Part model, mm, in its own coordinate system. A direction names the side the tool comes from. Give positions to 0.01 mm unless a question says otherwise; leave off trailing zeros. Order: outer loops, then holes, each group sorted by start corner. A loop starts at its lowest first (then second) coordinate and runs counter-clockwise, first axis right, second up. Notation, with made-up numbers: M 34.5,81 L 88.5,81 A32 cw 88.5,110 Z; hole C 33.25,19 d1. An arc over 180 degrees is marked long. Write each question's results on one line, items separated by ' | '. Start each with the question number.
from build123d import *

# Parameters (mm, degrees)
SKETCH1_R           = 5
BOSS_EXTRUDE1_DEPTH = 10
BOSS_EXTRUDE2_DEPTH = 10
SKETCH3_W           = 20
SKETCH3_H           = 20
SKETCH3_W_2         = 15
SKETCH3_H_2         = 15
BOSS_EXTRUDE3_DEPTH = 21
SKETCH4_W           = 50
SKETCH4_H           = 50
BOSS_EXTRUDE4_DEPTH = 3
SKETCH5_R           = 22.5
BOSS_EXTRUDE5_DEPTH = 75
SKETCH6_W           = 104.673759345
SKETCH6_H           = 11.076222709
BOSS_EXTRUDE6_DEPTH = 10


with BuildPart() as part:
    # Sketch1 → Boss-Extrude1 (new body)
    with BuildSketch(Plane(origin=(0, 0, 0), x_dir=(1, 0, 0), z_dir=(0, 1, 0))):
        with BuildLine():
            Line((0, 0), (30.876052193, 0))
            Line((30.876052193, 0), (30.876052193, -11.362717468))
            ThreePointArc((30.876052193, -11.362717468), (46.762190972, -21.786248919), (50, -3.063642105))
            Line((50, -3.063642105), (50, 0))
            Line((50, 0), (50, 50))
            Line((50, 50), (0, 50))
            Line((0, 50), (0, 0))
        make_face()
        with Locations(Location((42.238769661, -11.362717468, 0), (0, 0, 270))):
            Circle(SKETCH1_R, mode=Mode.SUBTRACT)
        with BuildLine():
            Line((9.874654059, 47.191553979), (24.296746366, 33.290272916))
            ThreePointArc((24.296746366, 33.290272916), (24.424993645, 26.799159409), (17.934255558, 26.653142217))
            Line((17.934255558, 26.653142217), (3.436266044, 40.475249935))
            ThreePointArc((3.436266044, 40.475249935), (3.288101967, 47.061421086), (9.874654059, 47.191553979))
        make_face(mode=Mode.SUBTRACT)
    extrude(amount=BOSS_EXTRUDE1_DEPTH)

    # Sketch2 → Boss-Extrude2 (add)
    with BuildSketch(Plane.XZ):
        Polygon((45, -5), (35, -5), (35, 0), (50, 0), (50, -15), (45, -15), align=None)
    extrude(amount=BOSS_EXTRUDE2_DEPTH)

    # Sketch3 → Boss-Extrude3 (add)
    with BuildSketch(Plane(origin=(0, 10, 0), x_dir=(1, 0, 0), z_dir=(0, 1, 0))):
        with Locations((10, 10)):
            Rectangle(SKETCH3_W, SKETCH3_H)
        with Locations((42.5, 42.5)):
            Rectangle(SKETCH3_W_2, SKETCH3_H_2)
    extrude(amount=BOSS_EXTRUDE3_DEPTH)

    # Sketch4 → Boss-Extrude4 (add)
    with BuildSketch(Plane(origin=(0, 31, 0), x_dir=(1, 0, 0), z_dir=(0, 1, 0))):
        with Locations((25, 25)):
            Rectangle(SKETCH4_W, SKETCH4_H)
    extrude(amount=BOSS_EXTRUDE4_DEPTH)

    # Sketch5 → Boss-Extrude5 (add)
    with BuildSketch(Plane(origin=(0, 34, 0), x_dir=(1, 0, 0), z_dir=(0, 1, 0))):
        with Locations(Location((25, 25, 0), (0, 0, 270))):
            Circle(SKETCH5_R)
    extrude(amount=BOSS_EXTRUDE5_DEPTH)

    # Sketch6 → Boss-Extrude6 (add)
    with BuildSketch(Plane(origin=(0, 109, 0), x_dir=(1, 0, 0), z_dir=(0, 1, 0))):
        with Locations((-23.301664344, 22.675113634)):
            Rectangle(SKETCH6_W, SKETCH6_H)
    extrude(amount=BOSS_EXTRUDE6_DEPTH)


solid = part.part
(1) Saw through at B-B on x = 13. Give the cut face in (y, z).
(2) Tool access for faces 4 (the flat face through (25, 31, -25)), 5 (the flat face through (16.985, 4.93, -40.338)), 6 (the flat face through (29.035, 114, -23)): list every direction of +Z, -Z, +X, -X, +Y, -Y with a clear straight run to the whole face (end or side of a thin tool).
(3) Saw through at C-C on x = -47. Give the cut face in (y, z), plus the area to 3 significant figures.
(4) Drop flat-ended pins along their axis: P1, Ø3, axis at x = 40, y = -4, coming from the -Z side; P2, Ø12, axis at y = 35.5, z = -38, coming from the -X side; P3, Ø11, axis at y = 112.5, z = -20.5, coming from the +X side; P4, Ø12, axis at x = -38.5, y = 99, coming from the -Z side. Give the stop position or say it passes through.
(5) Saw through at D-D on y = 62. Give the cut face in (x, z).
(6) Saw through at A-A on y = 28. Give the cut face in (x, z).
(7) Pull direction Z, two halves, no side cores. Call faces 1 (the flat face through (26, 0, -22)), 2 (the flat face through (40, -5, -5)), 3 (the cylindrical face through (24.49, 4.93, -26.87)): +Z half, -Z half, draft (parallel to the pull), parting line (faces both ways), or undercut.
(8) Probe L1, parallel to Y at x = 23, z = -2; L2, parallel to X at y = 8, z = -5.5; L3, parallel to Y at x = -46.5, z = -28. List the from-to ranges inside material, lowest first.
Taken from the geometry:
1) outline: M 0,-50 L 10,-50 L 10,-44.18 L 0,-44.18 Z; M 0,-31.36 L 10,-31.36 L 10,-20 L 31,-20 L 31,-50 L 34,-50 L 34,-44.03 L 109,-44.03 L 109,-28.21 L 119,-28.21 L 119,-17.14 L 109,-17.14 L 109,-5.97 L 34,-5.97 L 34,0 L 0,0 Z
2) face 4: none | face 5: -Y | face 6: +Z, -Z, +X, +Y
3) outline: M 109,-28.21 L 119,-28.21 L 119,-17.14 L 109,-17.14 Z | area: 111 mm²
4) P1: stops at z = -5 | P2: stops at x = 0 | P3: stops at x = 47.5 | P4: passes through
5) outline: C 25,-25 d45
6) outline: M 0,-20 L 20,-20 L 20,0 L 0,0 Z; M 35,-50 L 50,-50 L 50,-35 L 35,-35 Z
7) face 1: draft | face 2: -Z half | face 3: undercut
8) L1: y = 0 to 10, 31 to 34 | L2: x = 0 to 50 | L3: y = 109 to 119
